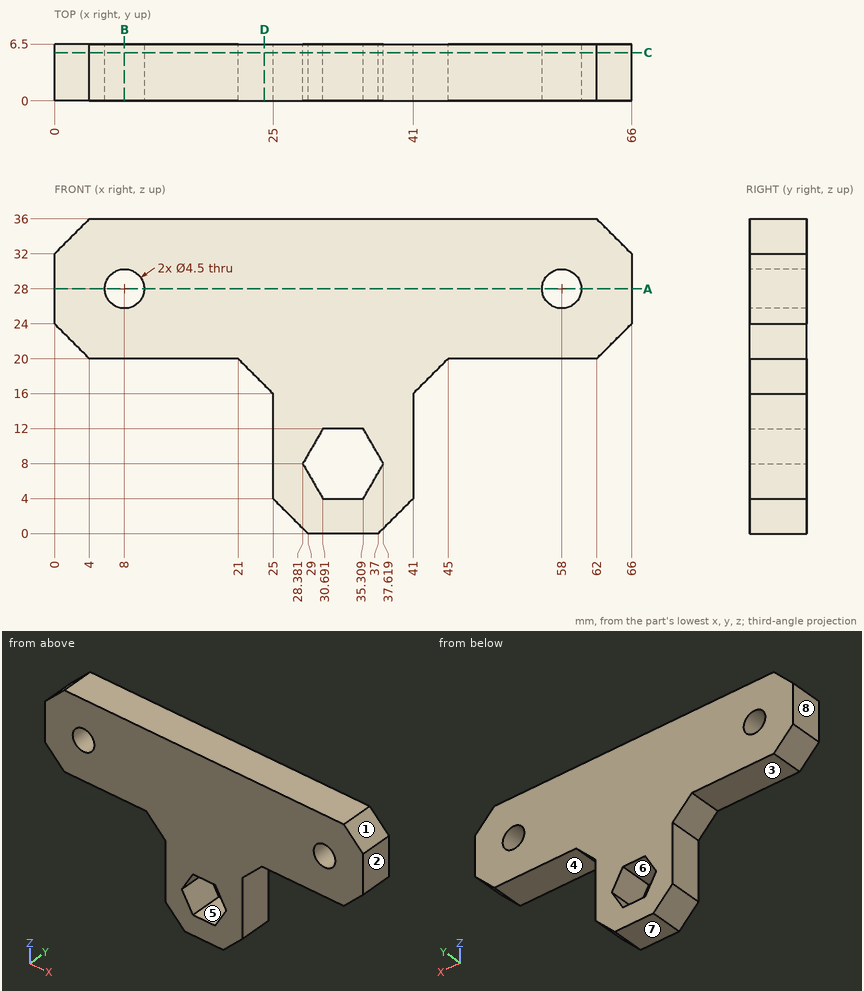
Can you work these out from the drawing? Everything is in mm from the part's minimum corner. A direction names the side the tool comes from. Coordinates: 2 decimals unless noted, no trailing zeros. Loops run counter-clockwise (first coordinate to the right, second up) from the corner with the lowest first, then second, coordinate; pieces in that order, holes last.
1) Please list where these lines run through material, in increasing order: line 1 along Z through (x, y) = (58, 3.5); line 2 along Z through (x, y) = (34, 1.5); line 3 along X through (y, z) = (5.5, 26).
Reported:
line 1: z = 20 to 25.75, 30.25 to 36
line 2: z = 0 to 4, 12 to 36
line 3: x = 0 to 6.97, 9.03 to 56.97, 59.03 to 66
2) Which directions (+Z, -Z, +X, -X, +Y, -Y) give clear straight access to the entire face, cutting with the end or side of a thin tool? Please do the marked faces 1, 2, 3, 4 and 5.
Reported:
face 1: +Z, +X, +Y, -Y
face 2: +Z, -Z, +X, +Y, -Y
face 3: -Z, -X, +Y, -Y
face 4: -Z, +X, +Y, -Y
face 5: +Y, -Y
3) Thinking about a two-plate mould opening in X: for the marked faces 6, 7 and 8, which applies, released by +X, released by -X, zero draft, split by the parting line, or undercut?
Reported:
face 6: undercut
face 7: zero draft
face 8: released by -X
4) Imagine slicing it at C-C (y = 5.5). List the corners of the cut face in (x, z) for me, and give its area (3 significant figures).
Reported:
outline: (0, 24) - (4, 20) - (21, 20) - (25, 16) - (25, 4) - (29, 0) - (37, 0) - (41, 4) - (41, 16) - (45, 20) - (62, 20) - (66, 24) - (66, 32) - (62, 36) - (4, 36) - (0, 32) - close; hole circle Ø4.5 at (8, 28); hole (28.38, 8) - (30.69, 4) - (35.31, 4) - (37.62, 8) - (35.31, 12) - (30.69, 12) - close; hole circle Ø4.5 at (58, 28)
area: 1,260 mm2
5) Imagine slicing it at D-D (x = 24). List the corners of the cut face in (y, z) for me.
Reported:
outline: (0, 17) - (6.5, 17) - (6.5, 36) - (0, 36) - close
6) Will these pins go through, and if not, where does the flat tip stop? pin 1 Ø1 at (x, y) = (24, 3.5) entering from -Z; pin 2 Ø3 at (x, y) = (13, 2) entering from -Z.
Reported:
pin 1: stops at z = 16.5
pin 2: stops at z = 20
7) Imagine slicing it at A-A (z = 28). List the corners of the cut face in (x, y) for me.
Reported:
outline: (0, 0) - (5.75, 0) - (5.75, 6.5) - (0, 6.5) - close; (10.25, 0) - (55.75, 0) - (55.75, 6.5) - (10.25, 6.5) - close; (60.25, 0) - (66, 0) - (66, 6.5) - (60.25, 6.5) - close
8) Imagine slicing it at B-B (x = 8). List the corners of the cut face in (y, z) for me.
Reported:
outline: (0, 20) - (6.5, 20) - (6.5, 25.75) - (0, 25.75) - close; (0, 30.25) - (6.5, 30.25) - (6.5, 36) - (0, 36) - close
